Print and shaded views of the part. All mm, measured from the part's lowest x, y and z. A direction names the side the tool comes from. Coordinates: 2 decimals unless noted, no trailing zeros. Loops run counter-clockwise (first coordinate to the right, second up) from the corner with the lowest first, then second, coordinate; pieces in that order, holes last.
1) Which spindle directions (+Z, -Z, +X, -X, +Y, -Y) get a long thin tool onto all of the face, cutting with end or side? Do the marked faces 1 and 2. Say none if no direction does.
2) Saw through at A-A, the plane z = 4.75. Write the cut outline in (x, y).
3) Wall check: line 1 along X through (y, z) = (3.5, 3.75); line 2 along Z through (x, y) = (4.5, 4). Give the ranges that are in metal, low to high.
4) Saw through at B-B, the plane y = 5.25. Write the cut outline in (x, z), and give its area (3 significant figures).
5) Pin check, flat tip, straight feed: pin 1 Ø4 at (y, z) = (7, 6) entering from -X. Stop position of the tip, or through.
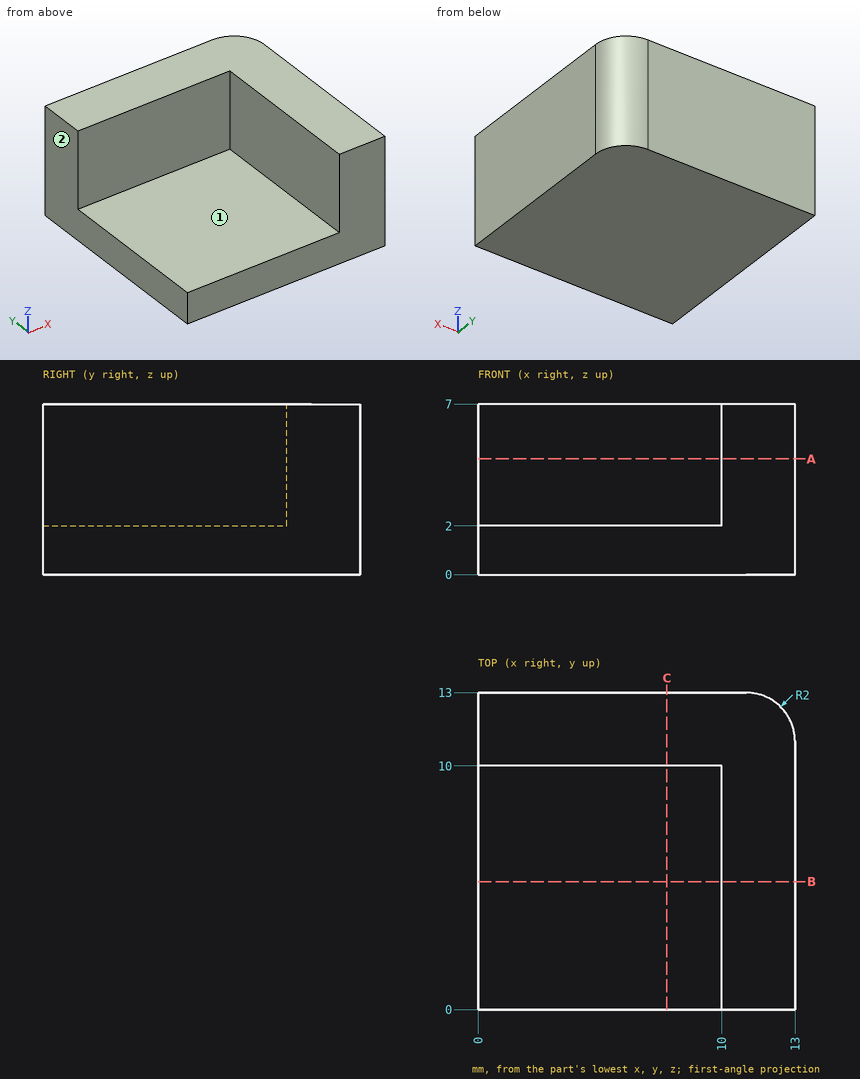
Data:
1. face 1: +Z, -X, -Y
1. face 2: +Z, -Z, -X, +Y, -Y
2. outline: (0, 10) - (10, 10) - (10, 0) - (13, 0) - (13, 11) arc R2 ccw to (11, 13) - (0, 13) - close
3. line 1: x = 10 to 13
3. line 2: z = 0 to 2
4. outline: (0, 0) - (13, 0) - (13, 7) - (10, 7) - (10, 2) - (0, 2) - close
4. area: 41.0 mm2
5. pin 1: stops at x = 10
